Autodesk Inventor part; units mm, degrees
ref_plane "YZ Plane" through (0, 0, 0) normal (1, 0, 0) x (0, 1, 0)
ref_plane "XZ Plane" through (0, 0, 0) normal (0, 1, 0) x (-1, 0, 0)
ref_plane "XY Plane" through (0, 0, 0) normal (0, 0, 1) x (1, 0, 0)
sketch "草图1" plane through (0, 0, 0) normal (0, 0, 1) x (1, 0, 0)
  circle A0 centre (0, 0) radius 4.5
  dimension "d0" = 9
extrude "拉伸1" add sketch "草图1" along normal blind 1
sketch "草图2" plane through (0, 0, 1) normal (0, 0, 1) x (1, 0, 0)
  line L0 (1.7321, -3) -> (-1.7321, -3)
  line L1 (-1.7321, -3) -> (-3.4641, 0)
  line L2 (-3.4641, 0) -> (-1.7321, 3)
  line L3 (-1.7321, 3) -> (1.7321, 3)
  line L4 (1.7321, 3) -> (3.4641, 0)
  line L5 (3.4641, 0) -> (1.7321, -3)
  line L6 (0, 0) -> (0, 0.7282)
  point P0 (0, 3)
  dimension "d3" = 0.7282
  dimension "d4" = 6
extrude "拉伸2" add sketch "草图2" along normal blind 4
sketch "草图3" plane through (0, 0, 0) normal (0, 0, -1) x (-1, 0, 0)
  circle A0 centre (0, 0) radius 2.5
  dimension "d7" = 5
extrude "拉伸3" add sketch "草图3" along normal blind 15
thread "螺纹1"
chamfer "倒角1" distance 0.25 angle 45 1 edges at (2.5, 0, -15)
fillet "圆角1" radius 0.25 1 edges at (-4.5, 0, 1)
fillet "圆角2" radius 0.25 6 edges at (0, -3, 5) (2.5981, -1.5, 5) (2.5981, 1.5, 5) (0, 3, 5) (-2.5981, 1.5, 5) (-2.5981, -1.5, 5)
properties part number "砂轮架带动曲柄轴盖螺丝"
The listing builds one solid part. Answer for the finished solid, in the listing's coordinates (mm). A direction names the side the tool comes from. Coordinates: 2 decimals unless noted, no trailing zeros. Loops run counter-clockwise (first coordinate to the right, second up) from the corner with the lowest first, then second, coordinate; pieces in that order, holes last. Notation, with made-up numbers: (4.5, 52.25) -> (62.5, 52.25) arc R31 ccw to (62.5, 81.25) -> close; hole circle Ø3 at (2, 40.5). An arc over 180 degrees is marked (long way). Write item = value, one per line. Start each with the question number.
1) A cutting plane is placed at A-A (x = 0). Give the vertices of the cut face in (y, z), then the cut area to 3 significant figures.
2) Straight lines are drawn through the part: line 1 (Z direction, x = 3.25, y = 0.75); line 2 (Y direction, x = 0, z = 2.75); line 3 (Y direction, x = -0.25, z = -5.5). For each, find the intervals that lie inside material, in ascending order. Write a range as from..to.
3) Given pin 1 Ø3 at (y, z) = (3, -10) entering from +X; pin 2 Ø1 at (x, z) = (-0.5, 2) entering from -Y; pin 3 Ø1 at (x, z) = (0, 3.5) entering from +Y, each flat-ended and moving along its own axis, determine where each tip first touches the part or whether it passes through.
4) A cutting plane is placed at B-B (z = -6.75). Give the vertices of the cut face in (x, y).
5) A tool of negligible diameter and unlimited length cuts with its end or side. For faces 1 (the face through (-2.6, -1.5, 2.8)), 2 (the face through (0, 3, 3)), 3 (the face through (0.54, 2.44, -7.27)), from which of +Z, -Z, +X, -X, +Y, -Y can it reach the whole face along a straight path? Write none if from no direction.
Responses:
q1.outline = (-4.5, 0) -> (-2.5, 0) -> (-2.5, -14.75) -> (-2.25, -15) -> (2.25, -15) -> (2.5, -14.75) -> (2.5, 0) -> (4.5, 0) -> (4.5, 0.75) arc R0.25 ccw to (4.25, 1) -> (3, 1) -> (3, 4.75) arc R0.25 ccw to (2.75, 5) -> (-2.75, 5) arc R0.25 ccw to (-3, 4.75) -> (-3, 1) -> (-4.25, 1) arc R0.25 ccw to (-4.5, 0.75) -> close
q1.area = 108 mm²
q2.line_1 = 0..1
q2.line_2 = -3..3
q2.line_3 = -2.49..2.49
q3.pin_1 = 2
q3.pin_2 = -3
q3.pin_3 = 3
q4.outline = circle Ø5 at (0, 0)
q5.face_1 = +Z, -X, -Y
q5.face_2 = +Z, +X, -X, +Y
q5.face_3 = -Z
